Design review of the part built by this model. Coordinates are the model's own, in mm. A direction names the side the tool comes from. Give positions to 0.01 mm unless a question says otherwise; leave off trailing zeros. Write each loop counter-clockwise with the first axis right and the second up, starting at its lowest first coordinate (ties: lowest second). Pieces come first, ordered by that corner, then holes. Notation, with made-up numbers: (9, 24) -> (39, 24) arc R24 cw to (39, 49) -> close; hole circle Ø9 at (-31.75, 86). An arc over 180 degrees is marked (long way). Use CSV: the item, a comma, the result in double quotes.
```python
from build123d import *

# Parameters (mm, degrees)
ESQUISSE1_W             = 100
ESQUISSE1_H             = 40
BOSS_EXTRU_1_DEPTH      = 6
ESQUISSE2_W             = 50
ESQUISSE2_H             = 6
BOSS_EXTRU_2_DEPTH      = 6
ENL_V_MAT_EXTRU_1_DEPTH = 47


with BuildPart() as part:
    # Esquisse1 → Boss.-Extru.1 (new body)
    with BuildSketch(Plane.XY):
        Rectangle(ESQUISSE1_W, ESQUISSE1_H)
    extrude(amount=BOSS_EXTRU_1_DEPTH)

    # Esquisse2 → Boss.-Extru.2 (add)
    with BuildSketch(Plane.XY.offset(6)):
        with Locations((0, 23)):
            Rectangle(ESQUISSE2_W, ESQUISSE2_H)
        with Locations((0, -23)):
            Rectangle(ESQUISSE2_W, ESQUISSE2_H)
    extrude(amount=-BOSS_EXTRU_2_DEPTH)

    # Esquisse3 → Enlèv. mat.-Extru.1 (cut, through all)
    with BuildSketch(Plane(origin=(0, 20, 0), x_dir=(1, 0, 0), z_dir=(0, 1, 0))):
        Polygon((-50, -6), (-37.5, 0), (-50, 0), align=None)
        Polygon((50, -6), (37.5, 0), (50, 0), align=None)
    extrude(amount=-ENL_V_MAT_EXTRU_1_DEPTH, mode=Mode.SUBTRACT)


solid = part.part
```
(1) For line 1 along Y through (x, z) = (-29.5, 3.5); line 2 along Z through (x, y) = (-40.5, 17); line 3 along X through (y, z) = (2, 4.25), list the stretches that pass through material, from the lowest coordinate up. Write a range as [from, to].
Established:
line 1,"y = [-20, 20]"
line 2,"z = [1.44, 6]"
line 3,"x = [-46.35, 46.35]"
(2) Take a section at C-C (y = -5.5). Write out the cut boundary in (x, z), then the cut area to 3 significant figures.
Established:
outline,"(-50, 6) -> (-37.5, 0) -> (37.5, 0) -> (50, 6) -> close"
area,"525 mm2"
(3) Take a section at A-A (z = 4.5). Write out the cut boundary in (x, y) (3 decimals), then the cut area to 3 significant figures.
Established:
outline,"(-46.875, -20) -> (-25, -20) -> (-25, -26) -> (25, -26) -> (25, -20) -> (46.875, -20) -> (46.875, 20) -> (25, 20) -> (25, 26) -> (-25, 26) -> (-25, 20) -> (-46.875, 20) -> close"
area,"4,350 mm2"
(4) Take a section at B-B (x = -39). Write out the cut boundary in (y, z), then the cut area to 3 significant figures.
Established:
outline,"(-20, 0.72) -> (20, 0.72) -> (20, 6) -> (-20, 6) -> close"
area,"211 mm2"
(5) Tool access review of faces 1 (the face through (-35, 20, 3)), 2 (the face through (35, -20, 3)), 3 (the face through (0, -26, 3)), 4 (the face through (25, 23, 3)), 5 (the face through (-35, -20, 3)): name each direction out of +Z, -Z, +X, -X, +Y, -Y from which nothing blocks a thin tool from reaching the whole face with its end or side.
Established:
face 1,"+Z, -Z, -X, +Y"
face 2,"+Z, -Z, +X, -Y"
face 3,"+Z, -Z, +X, -X, -Y"
face 4,"+Z, -Z, +X, +Y"
face 5,"+Z, -Z, -X, -Y"
(6) Clearance check with flat-ended pins moving along their axes: pin 1 (1.5 mm diameter, centred on y = 13, z = 3, fed in from -X); pin 2 (3 mm diameter, centred on x = -32.5, z = 2, fed in from -Y); pin 3 (3 mm diameter, centred on x = 36.5, z = 2, fed in from +Y). State where each tip first meets the part, or that it passes through.
Established:
pin 1,"stops at x = -45.31"
pin 2,"stops at y = -20"
pin 3,"stops at y = 20"
